from build123d import *

# Parameters (mm, degrees)
BOSS_EXTRUDE1_DEPTH              = 457.2
F_97_0_0059_DIAMETER_HOLE1_D     = 228.6
F_97_0_0059_DIAMETER_HOLE1_DEPTH = 228.601
CUT_EXTRUDE1_DEPTH               = 66.616681
CUT_EXTRUDE2_REACH               = 560.8


with BuildPart() as part:
    # Sketch1 → Boss-Extrude1 (new body, symmetric)
    with BuildSketch(Plane.XY):
        with BuildLine():
            Line((457.905011984, 152.4), (558.8, 152.4))
            Line((558.8, 152.4), (558.8, 482.6))
            Line((558.8, 482.6), (1270, 482.6))
            Line((1270, 482.6), (1270, 711.2))
            Line((1270, 711.2), (652.537814996, 711.2))
            ThreePointArc((652.537814996, 711.2), (0, 965.2), (-652.537814996, 711.2))
            Line((-652.537814996, 711.2), (-1270, 711.2))
            Line((-1270, 711.2), (-1270, 482.6))
            Line((-1270, 482.6), (-558.8, 482.6))
            Line((-558.8, 482.6), (-558.8, 152.4))
            Line((-558.8, 152.4), (-457.905011984, 152.4))
            ThreePointArc((-457.905011984, 152.4), (0, 482.6), (457.905011984, 152.4))
        make_face()
    extrude(amount=BOSS_EXTRUDE1_DEPTH, both=True)

    # #97 (0.0059) Diameter Hole1
    with Locations(Plane(origin=(0, 711.2, 0), x_dir=(1, 0, 0), z_dir=(0, 1, 0))):
        with Locations((-787.4, 0)):
            f_97_0_0059_diameter_hole1 = Hole(F_97_0_0059_DIAMETER_HOLE1_D / 2, depth=F_97_0_0059_DIAMETER_HOLE1_DEPTH)

    # Mirror7: #97 (0.0059) Diameter Hole1 across plane
    add(f_97_0_0059_diameter_hole1.mirror(Plane(origin=(0, 0, 0), x_dir=(0, 0, 1), z_dir=(1, 0, 0))), mode=Mode.SUBTRACT)

    # Sketch5 → Cut-Extrude1 (cut)
    with BuildSketch(Plane(origin=(0, 711.2, 0), x_dir=(1, 0, 0), z_dir=(0, 1, 0))):
        with BuildLine():
            Line((-652.537814996, 168.597156133), (-652.537814996, -168.597156133))
            ThreePointArc((-652.537814996, -168.597156133), (-571.5, 0), (-652.537814996, 168.597156133))
        make_face()
    cut_extrude1 = extrude(amount=CUT_EXTRUDE1_DEPTH, mode=Mode.SUBTRACT)

    # Mirror8: Cut-Extrude1 across plane
    add(cut_extrude1.mirror(Plane(origin=(0, 0, 0), x_dir=(0, 0, 1), z_dir=(1, 0, 0))), mode=Mode.SUBTRACT)

    # Sketch6 → Cut-Extrude2 (cut, up to next)
    with BuildSketch(Plane(origin=(0, 711.2, 0), x_dir=(1, 0, 0), z_dir=(0, 1, 0)), mode=Mode.PRIVATE) as cut_extrude2_sk1:
        with BuildLine():
            Line((-1130.228649433, 457.2), (-1270, 457.2))
            Line((-1270, 457.2), (-1270, -457.2))
            Line((-1270, -457.2), (-1130.228649433, -457.2))
            ThreePointArc((-1130.228649433, -457.2), (-1219.2, 0), (-1130.228649433, 457.2))
        make_face()
    cut_extrude2_tool1 = extrude(cut_extrude2_sk1.sketch, amount=-CUT_EXTRUDE2_REACH, mode=Mode.PRIVATE) & part.part
    add(cut_extrude2_tool1.solids().sort_by_distance((-1225.646525, 711.2, 0))[0], mode=Mode.SUBTRACT)
    # Sketch6 → Cut-Extrude2 (cut, up to next)
    with BuildSketch(Plane(origin=(0, 711.2, 0), x_dir=(1, 0, 0), z_dir=(0, 1, 0)), mode=Mode.PRIVATE) as cut_extrude2_sk2:
        with BuildLine():
            Line((1130.228649433, 457.2), (1270, 457.2))
            Line((1270, 457.2), (1270, -457.2))
            Line((1270, -457.2), (1130.228649433, -457.2))
            ThreePointArc((1130.228649433, -457.2), (1219.2, 0), (1130.228649433, 457.2))
        make_face()
    cut_extrude2_tool2 = extrude(cut_extrude2_sk2.sketch, amount=-CUT_EXTRUDE2_REACH, mode=Mode.PRIVATE) & part.part
    add(cut_extrude2_tool2.solids().sort_by_distance((1225.646525, 711.2, 0))[0], mode=Mode.SUBTRACT)

    # Sketch10 → CSK for M10 Flat Head Machine Screw1 (revolve, cut)
    with BuildSketch(Plane(origin=(0, 965.2, 0), x_dir=(0, 0, 1), z_dir=(1, 0, 0))):
        Polygon((0, 0), (0, 3060.754649308), (63.5, 3022.6), (63.5, 342.9), (76.2, 330.2), (76.2, 0), align=None)
    revolve(axis=Axis((0, 971.55, 0), (0, -1, 0)), mode=Mode.SUBTRACT)


solid = part.part
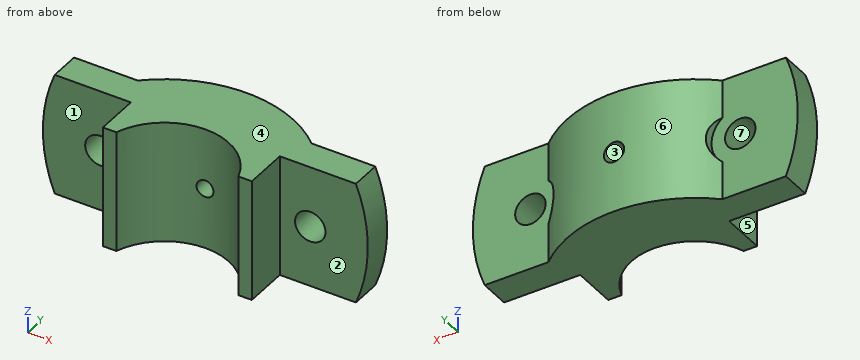
Input: part model. Units: mm. Frame: model coordinates. Face numbers are marked on the shaded views. A direction names the side the tool comes from. Coordinates: 2 decimals unless noted, no trailing zeros. Order: outer loops, then holes, each group sorted by start corner. A loop starts at its lowest first (then second) coordinate and runs counter-clockwise, first axis right, second up.
1. Draft query along X for the marked faces 4, 5, 6 and 7. Return one class per face: +X half, -X half, draft (parallel to the pull), parting line (faces both ways), or undercut.
Checked values:
face 4: draft
face 5: -X half
face 6: parting line
face 7: undercut
2. Cut plane D-D, the plane x = 0. Return loops of the section in (y, z), plus the area to 3 significant figures.
Checked values:
outline: (482.6, -457.2) - (965.2, -457.2) - (965.2, -76.2) - (635, -76.2) - (622.3, -63.5) - (482.6, -63.5) - close; (482.6, 63.5) - (622.3, 63.5) - (635, 76.2) - (965.2, 76.2) - (965.2, 457.2) - (482.6, 457.2) - close
area: 371,000 mm2
3. Cut plane C-C, the plane z = 287. Return loops of the section in (x, y).
Checked values:
outline: (-1184.94, 482.6) - (-558.8, 482.6) - (-558.8, 152.4) - (-457.91, 152.4) arc R482.6 cw to (457.91, 152.4) - (558.8, 152.4) - (558.8, 482.6) - (1184.94, 482.6) - (1184.94, 711.2) - (652.54, 711.2) arc R965.2 ccw to (-652.54, 711.2) - (-1184.94, 711.2) - close
4. Cut plane A-A, the plane x = 787.4. Return loops of the section in (y, z), plus the area to 3 significant figures.
Checked values:
outline: (482.6, -457.2) - (711.2, -457.2) - (711.2, -114.3) - (482.6, -114.3) - close; (482.6, 114.3) - (711.2, 114.3) - (711.2, 457.2) - (482.6, 457.2) - close
area: 157,000 mm2
5. Cut plane B-B, the plane y = 753.5. Return loops of the section in (x, z).
Checked values:
outline: (-603.2, -457.2) - (603.2, -457.2) - (603.2, -112.62) arc R215.9 cw to (603.2, 112.62) - (603.2, 457.2) - (-603.2, 457.2) - (-603.2, 112.62) arc R215.9 cw to (-603.2, -112.62) - close; hole circle Ø152.4 at (0, 0)
6. Ray query, line 1 along Z through (x, y) = (0, 508); line 2 along Z through (x, y) = (0, 860.5); line 3 along Y through (x, z) = (-596.5, 86.5). Return the intervals inside material, ascending.
Checked values:
line 1: z = -457.2 to -63.5, 63.5 to 457.2
line 2: z = -457.2 to -76.2, 76.2 to 457.2
line 3: y = 482.6 to 711.2
7. Contact query for flat-ended pins moving along their axis: P1, Ø6, axis at y = 673, z = -107, coming from the -X side; P2, Ø10, axis at x = 628, z = 283, coming from the +Y side; P3, Ø3, axis at x = -570.5, z = 63.5, coming from the -Y side. Output: stop coordinate, or through.
Checked values:
P1: stops at x = -1214.76
P2: stops at y = 737.21
P3: stops at y = 482.6
8. Access query for the marked faces 1, 2 and 3. Directions: +Z, -Z, +X, -X, +Y, -Y. A direction counts if a zero-diameter tool reaches every point of the face in a straight line with its end or side. Return the directions, or none.
Checked values:
face 1: +Z, -Z, -X, -Y
face 2: +Z, -Z, +X, -Y
face 3: +Y
